Part model, mm, in its own coordinate system. A direction names the side the tool comes from. Coordinates: 2 decimals unless noted, no trailing zeros. Loops run counter-clockwise (first coordinate to the right, second up) from the corner with the lowest first, then second, coordinate; pieces in that order, holes last. Notation, with made-up numbers: (33.5, 78) -> (80.5, 78) arc R22 cw to (80.5, 100) -> close; hole circle Ø3 at (88.25, 66.25). An arc over 180 degrees is marked (long way). Use one line per item in the form item = value. Start each with the question number.
(1) Mould opens along Y. For faces 1 (the cylindrical face through (-7.419, -1.382, 6.223)), 2 (the flat face through (-6.584, 0, 0)), 3 (the flat face through (20, 0, 0)), 4 (the flat face through (-4.057, 4.19, 7.396)) say: +Y half, -Y half, draft (parallel to the pull), parting line (faces both ways), or undercut.
(2) Drill centre lines: L1, parallel to Y at x = -6.95, z = 0 (3 decimals); L2, parallel to X at y = 5.25, z = -3.5; L3, parallel to X at y = -5.5, z = -5. Where is each one in solid material? Low to high. Write a range as [from, to].
(3) Pin check, flat tips, straight feed: P1, Ø8, axis at x = 11, y = -6, coming from the -Z side; P2, Ø5, axis at x = 3, z = -2, coming from the -Y side; P3, Ø4, axis at y = 2.5, z = -1, coming from the -X side. Stop position of each tip, or through.
(4) Band-saw the part on A-A on x = 7.75. Give the cut face in (y, z).
(5) 3-axis set-ups, long thin cutter, end or side, ignore diameter. For faces 5 (the cylindrical face through (10.06, -1.08, 4.88)), 6 (the flat face through (-4, -8.5, 0)): which of +Z, -Z, +X, -X, +Y, -Y reach the whole face in a straight line?
Autodesk Inventor part; units mm, degrees
ref_plane "Work Plane1" through (3, 0, 0) normal (0, 0.5, 0.866) x (1, 0, 0)
ref_plane "YZ Plane" through (0, 0, 0) normal (1, 0, 0) x (0, 1, 0)
ref_plane "XZ Plane" through (0, 0, 0) normal (0, 1, 0) x (-1, 0, 0)
sketch "Sketch1" plane through (0, 0, 0) normal (0, 0, 1) x (1, 0, 0)
  line L0 (0, 5) -> (0, 0)
  line L1 (0, 0) -> (20, 0)
  line L2 (20, 0) -> (20, 5)
  line L3 (20, 5) -> (0, 5)
  line L4 (-4, 0) -> (24, 0)
  line L5 (0, -1) -> (0, 6)
  dimension "d0" = 10
  dimension "d1" = 20
revolve "Body" add sketch "Sketch1" angle 360 about axis through (0, 0, 0) along (1, 0, 0)
sketch "Sketch2" plane through (0, 0, 0) normal (1, 0, 0) x (0, 1, 0)
  line L0 (0, 9.815) -> (8.5, 4.9075)
  line L1 (8.5, 4.9075) -> (8.5, -4.9075)
  line L2 (8.5, -4.9075) -> (0, -9.815)
  line L3 (0, -9.815) -> (-8.5, -4.9075)
  line L4 (-8.5, -4.9075) -> (-8.5, 4.9075)
  line L5 (-8.5, 4.9075) -> (0, 9.815)
  line L6 (-11.9, 0) -> (11.9, 0)
  line L7 (0, -13.7409) -> (0, 13.7409)
  point P0 (0, 0)
  point P1 (0, 0)
  dimension "d2" = 17
extrude "Head" add sketch "Sketch2" against normal blind 8.23
sketch "Sketch3" plane through (-8.23, 0, 0) normal (-1, 0, 0) x (0, 1, 0)
  circle A0 centre (0, 0) radius 6.375
  point P0 (0, 0)
  dimension "d12" = 12.75
extrude "Indent1" cut sketch "Sketch3" against normal blind 1.646
sketch "Sketch4" plane through (0, 0, 0) normal (0, 0, 1) x (1, 0, 0)
  line L0 (-8.23, 9.815) -> (-8.23, 8.5)
  line L1 (-8.23, 8.5) -> (-7.4708, 9.815)
  line L2 (-7.4708, 9.815) -> (-8.23, 9.815)
  line L3 (0, 9.815) -> (0, 8.5)
  line L4 (0, 8.5) -> (-0.7592, 9.815)
  line L5 (-0.7592, 9.815) -> (0, 9.815)
  line L6 (0, 0) -> (-8.23, 0)
  line L7 (-8.23, 0) -> (-8.23, 8.5)
  line L8 (0, 0) -> (0, 8.5)
  line L9 (-9.876, 0) -> (1.646, 0)
  line L10 (-7.4708, 9.815) -> (-0.7592, 9.815) construction
  line L11 (0, -1.963) -> (0, 11.7779)
  dimension "d6" = 30
  dimension "d7" = 30
  dimension "d16" = 17
  dimension "d17" = 17
  dimension "d18" = 19.6299
revolve "Chamfer1" cut sketch "Sketch4" angle 360 about axis through (-10, 0, 0) along (1, 0, 0)
fillet "Fillet1" radius 0.4 1 edges at (0, -5, 0)
thread "Thread"
ref_plane "Work Plane1" through (3, 0, 0) normal (0, 0.5, 0.866) x (1, 0, 0)
equation "\"d0\" = GD"
equation "\"d1\" = NLG"
equation "\"d2\" = SW"
equation "\"d3\" = KOH"
equation "\"d12\" = 0.75 * SW0"
equation "\"d14\" = 0.2 * KOH"
equation "\"d6\" = ANG1"
equation "\"d7\" = ANG1"
equation "\"d16\" = SW0"
equation "\"d17\" = SW0"
equation "\"d18\" = 1.1547 * SW"
equation "\"d11\" = RR"
equation "\"d8\" = GEL"
equation "\"NLG\" = 20"
equation "\"KOH\" = 8.23"
equation "\"GD\" = NND"
equation "\"GEL\" = 17"
equation "\"SW\" = 17"
equation "\"SW0\" = SW"
equation "\"ANG1\" = 30deg"
equation "\"RR\" = 0.4"
equation "\"GUL\" = 0.61345 * PTC"
equation "\"SPD\" = NND - 1.2269 * PTC"
equation "\"GD1\" = THREADDIA - 1.2269 * PTC"
equation "\"SDH\" = 11.2"
equation "\"TOA\" = 30deg"
equation "\"FAWI\" = 45deg"
equation "\"PTC\" = 1.5"
equation "\"GAL\" = 0.61345 * PTC"
equation "\"SD\" = 0"
equation "\"SD2\" = SDH"
equation "\"E0\" = 1.155 * SW"
properties part number "AS 1427 - M10 x 20" material "Steel, Mild"
A:
q1.face_1 = undercut
q1.face_2 = undercut
q1.face_3 = draft
q1.face_4 = +Y half
q2.L1 = [-8.5, -6.375], [6.375, 8.5]
q2.L2 = [-6.58, 0]
q2.L3 = [-8.23, 0]
q3.P1 = -4.58
q3.P2 = -5
q3.P3 = -6.58
q4.outline = circle Ø10 at (0, 0)
q5.face_5 = +X
q5.face_6 = +Z, -Z, +X, -X, -Y
